The model under review builds one solid part; all positions refer to its coordinate system, in mm. A direction names the side the tool comes from. Give positions to 0.01 mm unless a question says otherwise; leave off trailing zeros. Order: outer loops, then holes, each group sorted by start corner. A loop starts at its lowest first (then second) coordinate and runs counter-clockwise, first axis right, second up. Notation, with made-up numbers: (79, 68.5) - (108, 68.5) arc R23 ccw to (108, 91.5) - close; hole circle Ø4 at (5.25, 52). An arc over 180 degrees is marked (long way). Put each result on its own line as item: value.
```python
from build123d import *

# Parameters (mm, degrees)
EXTRUDE_1_DEPTH          = 150
EXTRUDE_2_DEPTH          = 150
CUT_EXTRUDE_3_DEPTH      = 161
CHAMFER_4_SIZE           = 10
CHAMFER_5_SIZE           = 10
EXTRUDE_7_DEPTH          = 20
CHAMFER_6_SIZE           = 5
CHAMFER_7_SIZE           = 5
EXTRUDE_8_DEPTH          = 58
EXTRUDE_8_DEPTH_BACK     = 60
EXTRUDE_9_DEPTH          = 20
EXTRUDE_17_DEPTH         = 20
EXTRUDE_17_DEPTH_BACK    = 1
CUT_EXTRUDE_6_DEPTH      = 276.322275262
CUT_EXTRUDE_6_DEPTH_BACK = 276.322275262
SKETCH_13_R              = 10
CUT_EXTRUDE_8_DEPTH      = 10
CUT_EXTRUDE_8_DEPTH_BACK = 10
CUT_EXTRUDE_9_DEPTH      = 31
CUT_EXTRUDE_9_DEPTH_BACK = 182


with BuildPart() as part:
    # 草图1 → 凸台-拉伸1 (new body)
    with BuildSketch(Plane(origin=(0, 0, 0), x_dir=(1, 0, 0), z_dir=(0, 1, 0))):
        Polygon((0, 0), (0, 110), (10, 110), (10, -10), (-110, -10), (-110, 0), align=None)
    extrude(amount=EXTRUDE_1_DEPTH)

    # 草图2 → 凸台-拉伸2 (add)
    with BuildSketch(Plane(origin=(0, 150, 0), x_dir=(1, 0, 0), z_dir=(0, 1, 0))):
        Polygon((10, 86.03773993), (10, -10), (58.018869965, 38.018869965), align=None)
        Polygon((-86.03773993, -10), (10, -10), (-38.018869965, -58.018869965), align=None)
    extrude(amount=-EXTRUDE_2_DEPTH)

    # 草图5 → 切除-拉伸3 (cut)
    with BuildSketch(Plane(origin=(0, 150, 0), x_dir=(1, 0, 0), z_dir=(0, 1, 0))):
        with BuildLine():
            Line((-86.03773993, -10), (-38.018869965, -58.018869965))
            Line((-38.018869965, -58.018869965), (-30.947802153, -50.947802153))
            ThreePointArc((-30.947802153, -50.947802153), (-59.992139056, -32.491105573), (-86.03773993, -10))
        make_face()
        with BuildLine():
            Line((10, 86.03773993), (58.018869965, 38.018869965))
            Line((58.018869965, 38.018869965), (50.947802153, 30.947802153))
            ThreePointArc((50.947802153, 30.947802153), (32.491105573, 59.992139056), (10, 86.03773993))
        make_face()
    extrude(amount=-CUT_EXTRUDE_3_DEPTH, mode=Mode.SUBTRACT)

    # 倒角4
    # the kernel refuses this chamfer: 10 mm, written as the material it adds along each edge
    with BuildSketch(Plane(origin=(-86.03773993, 150, 10), x_dir=(-1, 0, 0), z_dir=(0, -1, 0))) as chamfer_4_piece_1:
        with BuildLine():
            Line((CHAMFER_4_SIZE, 0), (-7.644165176, -7.308452513))
            ThreePointArc((-7.644165176, -7.308452513), (-3.915956427, -3.825991439), (0, 0))
            Line((0, 0), (CHAMFER_4_SIZE, 0))
        make_face()
    extrude(amount=150)

    # 倒角5
    # the kernel refuses this chamfer: 10 mm, written as the material it adds along each edge
    with BuildSketch(Plane(origin=(10, 150, -86.03773993), x_dir=(0.6910568330345163, 0, 0.7228004244024105), z_dir=(0, -1, 0))) as chamfer_5_piece_1:
        with BuildLine():
            Line((10.575761882, 0), (-CHAMFER_5_SIZE * 0.722800424402, -CHAMFER_5_SIZE * 0.691056833035))
            Line((-CHAMFER_5_SIZE * 0.722800424402, -CHAMFER_5_SIZE * 0.691056833035), (0, 0))
            ThreePointArc((0, 0), (5.474432495, -0.059279789), (10.575761882, 0))
        make_face()
    extrude(amount=150)

    # 草图8 → 凸台-拉伸7 (add)
    with BuildSketch(Plane(origin=(0, 0, 0), x_dir=(-1, 0, 0), z_dir=(0, -1, 0))):
        Polygon((110, 0), (0, 0), (0, 110), (-10, 110), (-133.743686708, -13.743686708), (-73.743686708, -73.743686708), (-13.743686708, -133.743686708), (110, -10), align=None)
    extrude(amount=EXTRUDE_7_DEPTH)

    # 倒角6
    chamfer_6_edges = [part.edges().sort_by_distance(p)[0] for p in [
        (-48.128156646, 0, 71.871843354),
    ]]
    chamfer(chamfer_6_edges, length=CHAMFER_6_SIZE)

    # 倒角7
    chamfer_7_edges = [part.edges().sort_by_distance(p)[0] for p in [
        (71.871843354, 0, -48.128156646),
    ]]
    chamfer(chamfer_7_edges, length=CHAMFER_7_SIZE)

    # 草图9 → 凸台-拉伸8 (add, two sides: drawn at the far end of the back side and taken through both)
    with BuildSketch(Plane(origin=(-0.289162235, 0, 0.289162235), x_dir=(0.7071067811865451, 0, 0.70710678118655), z_dir=(-0.70710678118655, 0, 0.7071067811865451)).offset(-EXTRUDE_8_DEPTH_BACK)):
        Polygon((14.142135624, 150), (67.756418231, 0), (14.142135624, 0), align=None)
    extrude(amount=EXTRUDE_8_DEPTH + EXTRUDE_8_DEPTH_BACK)

    # 草图10 → 凸台-拉伸9 (add)
    with BuildSketch(Plane(origin=(-40.947802153, 0, 40.947802153), x_dir=(0.7071067811865452, 0, 0.7071067811865498), z_dir=(-0.7071067811865498, 0, 0.7071067811865452))):
        with BuildLine():
            Line((14.142135624, 150), (87.333768107, 126.556202944))
            ThreePointArc((87.333768107, 126.556202944), (97.811967476, 112.737019173), (98.011481853, 95.395661207))
            Line((98.011481853, 95.395661207), (67.756418231, 0))
            Line((67.756418231, 0), (14.142135624, 150))
        make_face()
    extrude(amount=-EXTRUDE_9_DEPTH)

    # 草图12 → 凸台-拉伸17 (add, two sides: drawn at the far end of the back side and taken through both)
    with BuildSketch(Plane(origin=(40.947802153, 0, -40.947802153), x_dir=(0.7071067811865452, 0, 0.7071067811865498), z_dir=(-0.7071067811865498, 0, 0.7071067811865452)).offset(-EXTRUDE_17_DEPTH_BACK)):
        with BuildLine():
            Line((14.142135624, 150), (87.333768107, 126.556202944))
            ThreePointArc((87.333768107, 126.556202944), (97.811967476, 112.737019173), (98.011481853, 95.395661207))
            Line((98.011481853, 95.395661207), (67.756418231, 0))
            Line((67.756418231, 0), (14.142135624, 150))
        make_face()
    extrude(amount=EXTRUDE_17_DEPTH + EXTRUDE_17_DEPTH_BACK)

    # 草图13 → 切除-拉伸6 (cut, two sides: drawn at the far end of the back side and taken through both)
    with BuildSketch(Plane(origin=(-40.947802153, 0, 40.947802153), x_dir=(0.7071067811865452, 0, 0.7071067811865498), z_dir=(-0.7071067811865498, 0, 0.7071067811865452)).offset(-CUT_EXTRUDE_6_DEPTH_BACK)):
        with Locations((77.042401388, 104.51514855)):
            Circle(SKETCH_13_R)
    extrude(amount=CUT_EXTRUDE_6_DEPTH + CUT_EXTRUDE_6_DEPTH_BACK, mode=Mode.SUBTRACT)

    # 草图15 → 切除-拉伸8 (cut, two sides: drawn at the far end of the back side and taken through both)
    with BuildSketch(Plane(origin=(-0.289162235, 0, 0.289162235), x_dir=(0.7071067811865451, 0, 0.70710678118655), z_dir=(-0.70710678118655, 0, 0.7071067811865451)).offset(-CUT_EXTRUDE_8_DEPTH_BACK)):
        with BuildLine():
            Line((75.824326152, 0), (84.289321881, 0))
            ThreePointArc((84.289321881, 0), (93.528695136, -7.086316984), (104.289321881, -11.535004271))
            Line((104.289321881, -11.535004271), (104.289321881, -20))
            ThreePointArc((104.289321881, -20), (89.190074528, -11.233601025), (75.824326152, 0))
        make_face()
    extrude(amount=CUT_EXTRUDE_8_DEPTH + CUT_EXTRUDE_8_DEPTH_BACK, mode=Mode.SUBTRACT)

    # 草图18 → 切除-拉伸9 (cut, two sides: drawn at the far end of the back side and taken through both)
    with BuildSketch(Plane.XZ.offset(20).offset(-CUT_EXTRUDE_9_DEPTH_BACK)):
        Polygon((40.487345, 55.004008196), (-3.380540201, 10.938796408), (3.780279879, 3.810042897), (10.964971033, -3.294651596), (54.684805363, 40.917454531), (47.574262823, 47.948826004), align=None)
    extrude(amount=CUT_EXTRUDE_9_DEPTH + CUT_EXTRUDE_9_DEPTH_BACK, mode=Mode.SUBTRACT)


solid = part.part
```
(1) For faces 1 (the flat face through (5, 66, -110)), 2 (the cylindrical face through (63.018, -11.374, 63.399)), 3 (the flat face through (51.179, -9.56, 44.384)), 4 (the flat face through (69.26, -2.53, -47.25)), 5 (the flat face through (13.73, 92.72, 67.34)), list the 3-axis set-ups (+Z, -Z, +X, -X, +Y, -Y) from which the entire face can be reached by the end or side of a thin tool; tool diameter is ignored.
The answers:
face 1: -Z, +X, -X, +Y, -Y
face 2: none
face 3: +Y, -Y
face 4: -Z, +X, +Y
face 5: +X, +Y
(2) Clearance check with flat-ended pins moving along their axes: pin 1 Ø1 at (x, y) = (-69, 72.5) entering from -Z; pin 2 Ø10 at (y, z) = (16.5, 88.5) entering from +X; pin 3 Ø7 at (y, z) = (50, -101.5) entering from +X. State where each tip first meets the part, or that it passes through.
The answers:
pin 1: z = 0
pin 2: x = 20.2
pin 3: x = 10
(3) Take a section at C-C, the plane z = -65.5. Write out the cut boundary in (x, y), then the cut area to 3 significant figures.
The answers:
outline: (0, -20) - (54.5, -20) - (54.5, -5) - (47.43, 0) - (28.27, 0) - (28.27, 150) - (0, 150) - close
area: 5,310 mm^2
(4) The part is to be moulded in two halves that separate along X. For faces 6 (the flat face through (17.15, 76.05, 40.23)), 7 (the flat face through (-12.43, 76.05, 69.81)), 8 (the flat face through (41, -20, 10)), 9 (the flat face through (-20.5, 42.7, 62.1)), say which applies: pulls with the +X half, pulls with the -X half, needs draft (parallel to the pull), parting line crosses it, or undercut.
The answers:
face 6: undercut
face 7: undercut
face 8: needs draft
face 9: pulls with the -X half
(5) Wall thickness on L1, parallel to Z at x = 7.5, y = 59; L2, parallel to X at y = 110.5, z = 21.5; L3, parallel to Y at x = 89, z = 30.5: over which ranges is each line inside the solid? List them lowest first.
The answers:
L1: -110 to 0.13, 21.87 to 58.5, 61.11 to 89.4
L2: -73.68 to 7.13, 75.11 to 76.12, 98.78 to 104.81
L3: -20 to 0, 52.79 to 97.85, 111.18 to 127.46
(6) Take a section at B-B, the plane y = 36.5. Write out the cut boundary in (x, z).
The answers:
outline: (-110, 0) - (0, 0) - (0, -110) - (10, -110) - (10, -96.04) - (17.31, -78.39) arc R235.58 ccw to (50.95, -30.95) - (52.14, -32.14) - (80.82, -3.45) - (80.34, -2.97) - (97.75, 14.44) - (82.9, 29.29) - (65.49, 11.88) - (45.62, 31.75) - (10.96, -3.29) - (3.78, 3.81) - (-3.38, 10.94) - (31.45, 45.92) - (11.88, 65.49) - (29.29, 82.9) - (15.15, 97.04) - (-2.26, 79.63) - (-2.62, 79.99) - (-31.3, 51.3) - (-30.95, 50.95) arc R235.58 ccw to (-78.39, 17.31) - (-96.04, 10) - (-110, 10) - close
(7) Take a section at A-A, the plane x = -58. Write out the cut boundary in (y, z).
The answers:
outline: (-20, 0) - (150, 0) - (150, 33.96) - (0, 33.96) - (0, 54.93) - (-5, 62) - (-20, 62) - close
(8) Take a section at D-D, the plane y = 61.5. Write out the cut boundary in (x, z), then the cut area to 3 significant figures.
The answers:
outline: (-110, 0) - (0, 0) - (0, -110) - (10, -110) - (10, -96.04) - (17.31, -78.39) arc R235.58 ccw to (50.95, -30.95) - (52.14, -32.14) - (74.5, -9.77) - (74.02, -9.29) - (103.36, 20.05) - (88.51, 34.9) - (59.17, 5.56) - (39.34, 25.4) - (10.96, -3.29) - (3.78, 3.81) - (-3.38, 10.94) - (25.14, 39.59) - (5.56, 59.17) - (34.9, 88.51) - (20.76, 102.65) - (-8.58, 73.32) - (-8.93, 73.67) - (-31.3, 51.3) - (-30.95, 50.95) arc R235.58 ccw to (-78.39, 17.31) - (-96.04, 10) - (-110, 10) - close
area: 11,200 mm^2
